Part print with two shaded views. Sizes in mm from the minimum x, y, z corner. A direction names the side the tool comes from. Coordinates: 2 decimals unless noted, no trailing zeros. Write each loop counter-clockwise with the first axis right and the second up, starting at its lowest first coordinate (ties: lowest second). Pieces come first, ordered by that corner, then holes. Notation, with made-up numbers: M 16.5,-18.75 L 52.5,-18.75 A11 cw 52.5,-8.75 Z; hole C 30.25,61 d8. An arc over 180 degrees is marked long. Answer in a Markdown table with one row per item. Add a question column.
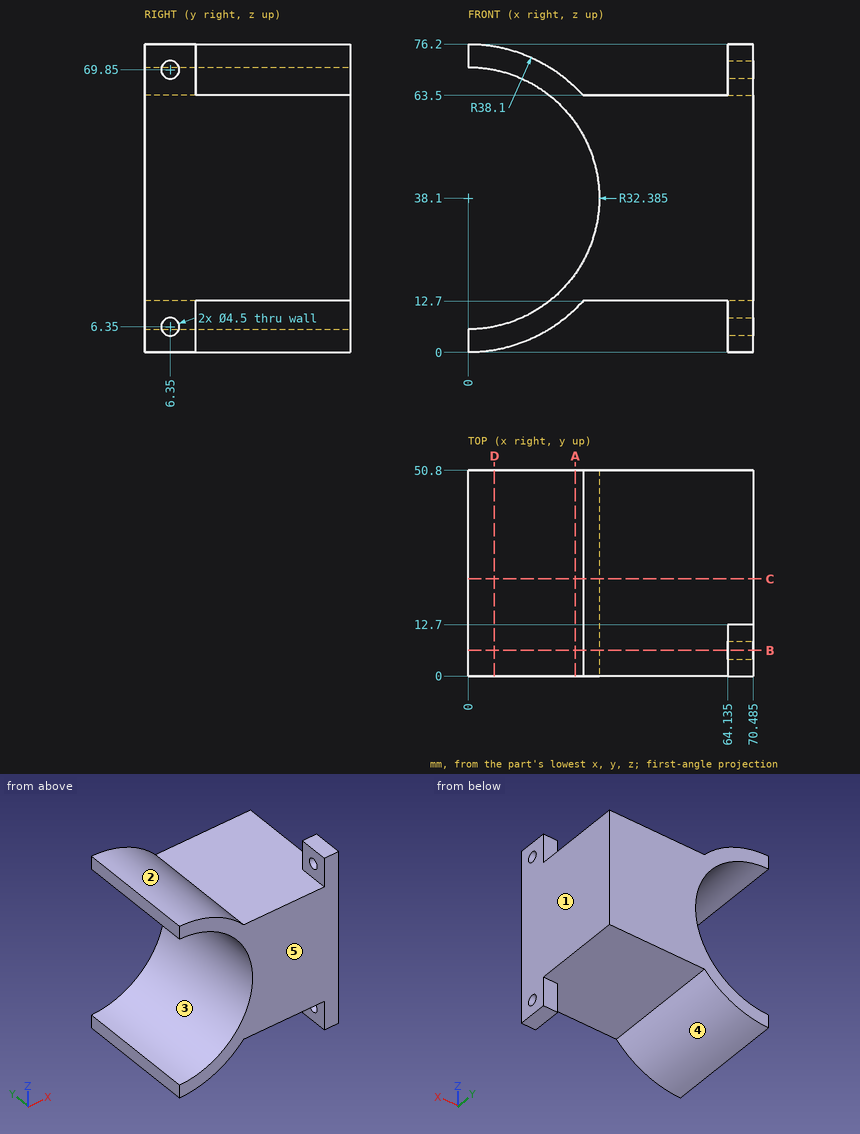
1) Slice it at A-A (x = 26.5). Give the cut face in (y, z).
2) Slice it at C-C (y = 24). Give the cut face in (x, z) (3 decimals), then the cut area to 3 significant figures.
3) Slice it at D-D (x = 6.5). Give the cut face in (y, z), then the cut area to 3 significant figures.
4) Drill centre lines: probe 1 along Y at (x, z) = (68.5, 69.85); probe 2 along Z at (x, y) = (66, 6); probe 3 along Z at (x, y) = (46, 29). Where is each one in solid material? Low to high.
5) Flat gauge pins, fed straight in: pin 1 Ø2 at (x, z) = (25.5, 11) entering from -Y; pin 2 Ø3 at (x, z) = (69, 8) entering from +Y; pin 3 Ø4 at (x, y) = (30, 44.5) entering from +Z; pin 4 Ø5 at (x, y) = (23, 33) entering from -Z. Where does each tip first touch, or does it go through?
6) Two-plate mould, pull along X, no slides. Class the marked faces 1, 2 and 3: released by +X, released by -X, zero draft, split by the parting line, or undercut.
7) Slice it at B-B (y = 6.35). Give the cut face in (x, z) (3 decimals), then the cut area to 3 significant figures.
8) Which spindle directions (+Z, -Z, +X, -X, +Y, -Y) get a long thin tool onto all of the face, cutting with end or side? Do the marked faces 4 and 5. Say none if no direction does.
Ans:
| question | item | result |
|---|---|---|
| 1 | outline | M 0,10.73 L 50.8,10.73 L 50.8,19.48 L 0,19.48 Z; M 0,56.72 L 50.8,56.72 L 50.8,65.47 L 0,65.47 Z |
| 2 | outline | M 0,0 A38.1 ccw 28.398,12.7 L 70.485,12.7 L 70.485,63.5 L 28.398,63.5 A38.1 ccw 0,76.2 L 0,70.485 A32.385 cw 0,5.715 Z |
| 2 | area | 2,430 mm2 |
| 3 | outline | M 0,0.56 L 50.8,0.56 L 50.8,6.37 L 0,6.37 Z; M 0,69.83 L 50.8,69.83 L 50.8,75.64 L 0,75.64 Z |
| 3 | area | 591 mm2 |
| 4 | probe 1 | y = 0 to 4.1, 8.6 to 12.7 |
| 4 | probe 2 | z = 0 to 4.13, 8.57 to 67.63, 72.07 to 76.2 |
| 4 | probe 3 | z = 12.7 to 63.5 |
| 5 | pin 1 | stops at y = 0 |
| 5 | pin 2 | stops at y = 12.7 |
| 5 | pin 3 | stops at z = 63.94 |
| 5 | pin 4 | stops at z = 5.99 |
| 6 | face 1 | released by +X |
| 6 | face 2 | undercut |
| 6 | face 3 | released by -X |
| 7 | outline | M 0,0 A38.1 ccw 28.398,12.7 L 64.135,12.7 L 64.135,8.6 L 70.485,8.6 L 70.485,67.6 L 64.135,67.6 L 64.135,63.5 L 28.398,63.5 A38.1 ccw 0,76.2 L 0,70.485 A32.385 cw 0,5.715 Z; M 64.135,0 L 70.485,0 L 70.485,4.1 L 64.135,4.1 Z; M 64.135,72.1 L 70.485,72.1 L 70.485,76.2 L 64.135,76.2 Z |
| 7 | area | 2,540 mm2 |
| 8 | face 4 | -Z, +Y, -Y |
| 8 | face 5 | +Z, -Z, +X, -X, -Y |
